Autodesk Inventor part; units mm, degrees
ref_plane "YZ Plane" through (0, 0, 0) normal (1, 0, 0) x (0, 1, 0)
ref_plane "XZ Plane" through (0, 0, 0) normal (0, 1, 0) x (-1, 0, 0)
ref_plane "XY Plane" through (0, 0, 0) normal (0, 0, 1) x (1, 0, 0)
sketch "Sketch1" plane through (0, 0, 0) normal (1, 0, 0) x (0, 1, 0)
  circle A0 centre (0, 0) radius 1.5
  circle A1 centre (0, 0) radius 3
  dimension "d0" = 3
  dimension "d1" = 6
extrude "Extrusion1" add sketch "Sketch1" against normal blind 16 contours A0
extrude "Extrusion2" add sketch "Sketch1" along normal blind 3 contours A0 | A1
sketch "Sketch2" plane through (3, 0, 0) normal (1, 0, 0) x (0, 0, -1)
  circle A0 centre (0, 0) radius 3
  circle A1 centre (0, 0) radius 3
  line L0 (-0.5749, -2.9444) -> (-0.5749, 2.9444)
  line L1 (0.5749, -2.9444) -> (0.5749, 2.9444)
  line L2 (0, 0) -> (0, 3)
extrude "Extrusion3" cut sketch "Sketch2" against normal blind 2 contours L1 A0 L0
chamfer "Chamfer1" distance 0.5 angle 45 1 edges at (-16, -1.5, 0)
thread "Thread2"
properties part number "screw_M3-10" material "Сталь, легированная"
Part model, mm, in its own coordinate system. A direction names the side the tool comes from. Give positions to 0.01 mm unless a question says otherwise; leave off trailing zeros. Write each loop counter-clockwise with the first axis right and the second up, starting at its lowest first coordinate (ties: lowest second). Pieces come first, ordered by that corner, then holes. Notation, with made-up numbers: M 7,59.25 L 58,59.25 A22 ccw 58,66.25 Z; hole C 11.5,-38 d11. An arc over 180 degrees is marked long. Use CSV: the item, a comma, the result in double quotes.
Item 1: Slice it at A-A on z = 0. Write the cut outline in (x, y), plus the area to 4 significant figures.
Taken from the geometry:
outline,"M -16,-1 L -15.5,-1.5 L 0,-1.5 L 0,-3 L 1,-3 L 1,3 L 0,3 L 0,1.5 L -15.5,1.5 L -16,1 Z"
area,"53.75 mm²"
Item 2: Slice it at D-D on y = 2.5. Write the cut outline in (x, z).
Taken from the geometry:
outline,"M 0,-1.66 L 3,-1.66 L 3,-0.57 L 1,-0.57 L 1,0.57 L 3,0.57 L 3,1.66 L 0,1.66 Z"
Item 3: Which spindle directions (+Z, -Z, +X, -X, +Y, -Y) get a long thin tool onto all of the face, cutting with end or side? Do faces 1 (the face through (2, 0, 0.575)), 2 (the face through (3, 0, -2)), 3 (the face through (-7.64, -1.5, 0.07)). Say none if no direction does.
Taken from the geometry:
face 1,"+X, +Y, -Y"
face 2,"+Z, -Z, +X, +Y, -Y"
face 3,"-X"
Item 4: Pull direction Z, two halves, no side cores. Call faces 4 (the face through (0, 1.3, -1.3)), 5 (the face through (2, 0, -0.575)), 6 (the face through (1.48, 2.77, 1.15)): +Z half, -Z half, draft (parallel to the pull), parting line (faces both ways), or undercut.
Taken from the geometry:
face 4,"draft"
face 5,"undercut"
face 6,"parting line"
Item 5: Pin check, flat tips, straight feed: P1, Ø0.6, axis at x = 2.5, y = 1, coming from the +Z side; P2, Ø3, axis at x = -1, z = 1, coming from the -Y side; P3, Ø0.6, axis at y = -0.5, z = 0, coming from the +X side; P4, Ø1.5, axis at x = -7, z = -0.5, coming from the +Y side. Stop position of each tip, or through.
Taken from the geometry:
P1,"stops at z = 2.92"
P2,"stops at y = -3"
P3,"stops at x = 1"
P4,"stops at y = 1.5"
Item 6: Drill centre lines: probe 1 along Z at (x, y) = (1.5, -2.6); probe 2 along X at (y, z) = (-1.9, -1.55); probe 3 along X at (y, z) = (0.8, -0.1). Where is each one in solid material? Low to high.
Taken from the geometry:
probe 1,"z = -1.5 to -0.57, 0.57 to 1.5"
probe 2,"x = 0 to 3"
probe 3,"x = -16 to 1"
Item 7: Slice it at B-B on y = 0. Write the cut outline in (x, z), plus the area to 3 significant figures.
Taken from the geometry:
outline,"M -16,-1 L -15.5,-1.5 L 0,-1.5 L 0,-3 L 3,-3 L 3,-0.57 L 1,-0.57 L 1,0.57 L 3,0.57 L 3,3 L 0,3 L 0,1.5 L -15.5,1.5 L -16,1 Z"
area,"63.5 mm²"
Item 8: Slice it at C-C on x = 0.25. Write the cut outline in (y, z).
Taken from the geometry:
outline,"C 0,0 d6"
